from build123d import *

# Parameters (mm, degrees)
SKETCH1_R           = 4
SKETCH1_R_2         = 2.5
BOSS_EXTRUDE1_DEPTH = 420
SKETCH1_3_R         = 6
SKETCH1_3_R_2       = 4
BOSS_EXTRUDE2_DEPTH = 414
SKETCH1_4_R         = 6
SKETCH1_4_R_2       = 4
CUT_EXTRUDE1_DEPTH  = 20
SKETCH1_5_R         = 4
SKETCH1_5_R_2       = 2.5
CUT_EXTRUDE2_DEPTH  = 10
CUT_EXTRUDE3_DEPTH  = 6


with BuildPart() as part:
    # Sketch1 → Boss-Extrude1 (new body)
    # profile 1 of 5: a face of its own
    with BuildSketch(Plane(origin=(0, 0, 0), x_dir=(1, 0, 0), z_dir=(0, 1, 0))):
        with Locations(Location((0, 0, 0), (0, 0, 270))):
            Circle(SKETCH1_R)
        Circle(SKETCH1_R_2, mode=Mode.SUBTRACT)
    # profile 2 of 5: a face of its own
    with BuildSketch(Plane(origin=(0, 0, 0), x_dir=(1, 0, 0), z_dir=(0, 1, 0))):
        with BuildLine():
            Line((1.5, -2), (1.5, 2))
            ThreePointArc((1.5, 2), (-2.5, 0), (1.5, -2))
        make_face()
    # profile 3 of 5: a face of its own
    with BuildSketch(Plane(origin=(0, 0, 0), x_dir=(1, 0, 0), z_dir=(0, 1, 0))):
        with BuildLine():
            ThreePointArc((2.5, 0), (2.236067977, 1.118033989), (1.5, 2))
            Line((1.5, 2), (1.5, -2))
            ThreePointArc((1.5, -2), (2.236067977, -1.118033989), (2.5, 0))
        make_face()
    # profile 4 of 5: a face of its own
    with BuildSketch(Plane(origin=(0, 0, 0), x_dir=(1, 0, 0), z_dir=(0, 1, 0))):
        with BuildLine():
            Line((1.5, -2), (1.5, 2))
            ThreePointArc((1.5, 2), (-2.5, 0), (1.5, -2))
        make_face()
    # profile 5 of 5: a face of its own
    with BuildSketch(Plane(origin=(0, 0, 0), x_dir=(1, 0, 0), z_dir=(0, 1, 0))):
        with BuildLine():
            ThreePointArc((2.5, 0), (2.236067977, 1.118033989), (1.5, 2))
            Line((1.5, 2), (1.5, -2))
            ThreePointArc((1.5, -2), (2.236067977, -1.118033989), (2.5, 0))
        make_face()
    extrude(amount=BOSS_EXTRUDE1_DEPTH)

    # Sketch1_3 → Boss-Extrude2 (add)
    with BuildSketch(Plane(origin=(0, 0, 0), x_dir=(1, 0, 0), z_dir=(0, 1, 0))):
        with Locations(Location((0, 0, 0), (0, 0, 270))):
            Circle(SKETCH1_3_R)
        with Locations(Location((0, 0, 0), (0, 0, 270))):
            Circle(SKETCH1_3_R_2, mode=Mode.SUBTRACT)
    extrude(amount=BOSS_EXTRUDE2_DEPTH)

    # Sketch1_4 → Cut-Extrude1 (cut)
    with BuildSketch(Plane(origin=(0, 0, 0), x_dir=(1, 0, 0), z_dir=(0, 1, 0))):
        with Locations(Location((0, 0, 0), (0, 0, 270))):
            Circle(SKETCH1_4_R)
        with Locations(Location((0, 0, 0), (0, 0, 270))):
            Circle(SKETCH1_4_R_2, mode=Mode.SUBTRACT)
    extrude(amount=CUT_EXTRUDE1_DEPTH, mode=Mode.SUBTRACT)

    # Sketch1_5 → Cut-Extrude2 (cut)
    with BuildSketch(Plane(origin=(0, 0, 0), x_dir=(1, 0, 0), z_dir=(0, 1, 0))):
        with Locations(Location((0, 0, 0), (0, 0, 270))):
            Circle(SKETCH1_5_R)
        with Locations(Location((0, 0, 0), (0, 0, 270))):
            Circle(SKETCH1_5_R_2, mode=Mode.SUBTRACT)
    extrude(amount=CUT_EXTRUDE2_DEPTH, mode=Mode.SUBTRACT)

    # Sketch1_6 → Cut-Extrude3 (cut)
    with BuildSketch(Plane(origin=(0, 0, 0), x_dir=(1, 0, 0), z_dir=(0, 1, 0))):
        Polygon((1.5, 33.931712199), (1.5, 2), (1.5, -2), (1.5, -33.931712199), (65.363424399, -33.931712199), (65.363424399, 33.931712199), align=None)
    extrude(amount=CUT_EXTRUDE3_DEPTH, mode=Mode.SUBTRACT)


solid = part.part
Geometry check sheet. Reference: the model listing, model coordinates, mm. A direction names the side the tool comes from. Give positions to 0.01 mm unless a question says otherwise; leave off trailing zeros. Loops run counter-clockwise (first coordinate to the right, second up) from the corner with the lowest first, then second, coordinate; pieces in that order, holes last. Notation, with made-up numbers: M 49.5,7.5 L 65.5,7.5 A6 cw 65.5,13.5 Z; hole C -10,53 d10. An arc over 180 degrees is marked long. Answer as a JSON object with one key per item and string values. Group by question number.
Item 1: Gauge pin test, flat ends, axial feed: pin 1 (3 mm diameter, centred on y = 2, z = 0, fed in from +X); pin 2 (0.5 mm diameter, centred on x = 2, z = -1, fed in from -Y); pin 3 (2 mm diameter, centred on x = -4.5, y = 164, fed in from +Z). Record the tip position at first contact, or that the pin passes through.
Item 2: Material ranges on L1, parallel to X at y = 299.5, z = 1; L2, parallel to X at y = 130, z = -0.25, recorded low to high.
Item 3: Access from +Z, -Z, +X, -X, +Y, -Y to the whole of each face (thin tool, end or side, straight path). Record for faces 1 (the flat face through (-3.92, 20, -1.42)), 2 (the flat face through (-3.92, 414, -1.42)), 3 (the cylindrical face through (1.802, 214.242, 5.723)).
Item 4: Sectioned sample at B-B on y = 375. Record the boundary of the cut face in (x, z), plus the area to 3 significant figures.
Item 5: Sectioned sample at A-A on z = 0. Record the boundary of the cut face in (x, y), plus the area to 3 significant figures.
Findings below:
{
 "1": {"pin 1": "x = 1.5", "pin 2": "y = 6", "pin 3": "z = 4.87"},
 "2": {"L1": "-5.92 to 5.92", "L2": "-5.99 to 5.99"},
 "3": {"face 1": "-Y", "face 2": "+Y", "face 3": "+Y, -Y"},
 "4": {"outline": "C 0,0 d12", "area": "113 mm2"},
 "5": {"outline": "M -6,20 L -4,20 L -4,10 L -2.5,10 L -2.5,0 L 1.5,0 L 1.5,6 L 2.5,6 L 2.5,10 L 4,10 L 4,20 L 6,20 L 6,414 L 4,414 L 4,420 L -4,420 L -4,414 L -6,414 Z", "area": "4,900 mm2"}
}
